The listing builds one solid part. Answer for the finished solid, in the listing's coordinates (mm). A direction names the side the tool comes from. Give positions to 0.01 mm unless a question says otherwise; leave off trailing zeros. Loops run counter-clockwise (first coordinate to the right, second up) from the corner with the lowest first, then second, coordinate; pieces in that order, holes last. Notation, with made-up numbers: (34.5, -39) - (52.5, -39) arc R12 ccw to (52.5, -20) - close; hole circle Ø2 at (34.5, 67.25). An arc over 180 degrees is marked (long way). One line per item, written item: value. Start each with the question number.
Autodesk Fusion 360 part; units mm, degrees
sketch "Sketch6" plane through (0, 0, 0) normal (0, 0, 1) x (1, 0, 0)
  line L0 (0, 0) -> (3, 0)
  line L1 (3, 0) -> (3, 26)
  line L2 (3, 26) -> (0, 26)
  line L3 (0, 26) -> (0, 0)
  dimension "d27" = 3
  dimension "d28" = 26
extrude "Extrude8" add sketch "Sketch6" along normal blind 3
sketch "Sketch7" plane through (0, 0, 0) normal (0, 1, 0) x (1, 0, 0)
sketch "Sketch8" plane through (0, 0, 0) normal (0, -1, 0) x (1, 0, 0)
  line L0 (0, 0) -> (3, 0)
  line L1 (3, 0) -> (3, 3)
  line L2 (3, 3) -> (0, 3)
  line L3 (0, 3) -> (0, 0)
  line L4 (3, 3) -> (0, 3)
  line L5 (0, 3) -> (0, 18.5)
  line L6 (0, 18.5) -> (3, 18.5)
  line L7 (3, 18.5) -> (3, 3)
  dimension "d31" = 3
  dimension "d32" = 15.5
extrude "Extrude9" add sketch "Sketch8" along normal blind 3
sketch "Sketch9" plane through (0, 26, 0) normal (0, 1, 0) x (-1, 0, 0)
  line L0 (-3, 0) -> (0, 0)
  line L1 (0, 0) -> (0, 3)
  line L2 (0, 3) -> (-3, 3)
  line L3 (-3, 3) -> (-3, 0)
  line L4 (0, 0) -> (-3, 0)
  line L5 (-3, 0) -> (-3, 18.5)
  line L6 (-3, 18.5) -> (0, 18.5)
  line L7 (0, 18.5) -> (0, 0)
  dimension "d35" = 3
  dimension "d36" = 18.5
extrude "Extrude10" add sketch "Sketch9" along normal blind 3
sketch "Sketch10" plane through (0, 0, 0) normal (0, 1, 0) x (-1, 0, 0)
  line L0 (-3, 3) -> (0, 3)
  line L1 (0, 3) -> (0, 18.5)
  line L2 (0, 18.5) -> (-3, 18.5)
  line L3 (-3, 18.5) -> (-3, 3)
  line L4 (-1.5, 18.5) -> (-1.5, 17)
  circle A0 centre (-1.5, 17) radius 1.5
  dimension "d39" = 1.5
  dimension "d40" = 3
sketch "Sketch12" plane through (0, 26, 0) normal (0, -1, 0) x (1, 0, 0)
  line L0 (0, 3) -> (3, 3)
  line L1 (3, 3) -> (3, 18.5)
  line L2 (3, 18.5) -> (0, 18.5)
  line L3 (0, 18.5) -> (0, 3)
  line L4 (1.5, 18.5) -> (1.5, 17.15)
  circle A0 centre (1.5, 17.15) radius 1.35
  dimension "d53" = 1.35
  dimension "d54" = 2.7
extrude "Extrude15" add sketch "Sketch12" along normal blind 5 contours A0
sketch "Sketch13" plane through (0, 0, 0) normal (0, 1, 0) x (-1, 0, 0)
  line L0 (-3, 3) -> (0, 3)
  line L1 (0, 3) -> (0, 18.5)
  line L2 (0, 18.5) -> (-3, 18.5)
  line L3 (-3, 18.5) -> (-3, 3)
  line L4 (-1.5, 18.5) -> (-1.5, 17.15)
  circle A0 centre (-1.5, 17.15) radius 1.35
  dimension "d57" = 1.35
  dimension "d58" = 2.7
extrude "Extrude16" add sketch "Sketch13" along normal blind 5 contours A0
fillet "Fillet4" radius 1.5 8 edges at (3, -1.5, 18.5) (1.5, -3, 18.5) (0, -1.5, 18.5) (1.5, 29, 18.5) (3, 27.5, 18.5) (0, 27.5, 18.5) (1.5, 29, 0) (1.5, -3, 0)
1. Determine the mould class of faces 1 (the flat face through (1, 21, 17)), 2 (the cylindrical face through (1.48, 28.57, 0.45)), 3 (the flat face through (1, 13, 0)) for opening direction Y: released by +Y, released by -Y, zero draft, split by the parting line, or undercut.
2. For faces 4 (the cylindrical face through (1.21, 23.54, 18.47)), 5 (the flat face through (2, 5, 17)), 6 (the flat face through (1, 13, 3)), 7 (the cylindrical face through (0.45, -1.19, 18.07)), determine the directions among +Z, -Z, +X, -X, +Y, -Y from which every point of the face is accessible in a straight line to the end or side of a thin tool.
3. A cutting plane is placed at C-C (y = 7). Determine the outline of the cut face in (x, z).
4. A cutting plane is placed at B-B (y = 25). Determine the outline of the cut face in (x, z), plus the area to 3 significant figures.
5. A cutting plane is placed at A-A (z = 11). Determine the outline of the cut face in (x, y), plus the area to 3 significant figures.
6. Find the intervals of material crossed by L1, parallel to Y at x = 1.65, z = 11; L2, parallel to Z at x = 1.4, y = 3; L3, parallel to Z at x = 1.9, y = 15.5, in increasing order. Write a range as [from, to].
7. A flat-ended cylindrical pin translates along its axis: pin 1 (1.5 mm diameter, centred on x = 2, y = 9, fed in from +Z). Find the tip coordinate at first contact, or state that the pin passes through.
Results below:
1. face 1: undercut
1. face 2: released by +Y
1. face 3: zero draft
2. face 4: none
2. face 5: +Z, +X, -X
2. face 6: +X, -X
2. face 7: +Z, -X, +Y, -Y
3. outline: (0, 0) - (3, 0) - (3, 3) - (0, 3) - close
4. outline: (0, 0) - (3, 0) - (3, 3) - (0, 3) - close; circle Ø2.7 at (1.5, 17.15)
4. area: 14.7 mm^2
5. outline: (0, -3) - (3, -3) - (3, 0) - (0, 0) - close; (0, 26) - (3, 26) - (3, 29) - (0, 29) - close
5. area: 18.0 mm^2
6. L1: y = [-3, 0], [26, 29]
6. L2: z = [0, 3], [15.8, 18.5]
6. L3: z = [0, 3]
7. pin 1: stops at z = 3
